Could you check a few things on this model? Use its own coordinates, in mm. Face numbers are marked on the shaded views. A direction names the side the tool comes from. Give positions to 0.01 mm unless a question says otherwise; leave off trailing zeros. Write each loop counter-clockwise with the first axis right and the second up, starting at its lowest first coordinate (ties: lowest second). Pieces come first, ordered by that corner, then holes. Notation, with made-up numbers: M -12.75,-30.5 L 3.25,-30.5 A22 cw 3.25,-5.5 Z; hole C -8.75,51 d8. An arc over 180 degrees is marked long. Use one line per item in the form item = value.
from build123d import *

# Parameters (mm, degrees)
F1_DEPTH = 63.5
F2_DEPTH = 25.4
F3_DEPTH = 7.9375
F5_R     = 6.35


with BuildPart() as f1:
    # F0 (on Front) → F1 (new body, symmetric)
    with BuildSketch(Plane.XZ):
        Polygon((22.225, 9.525), (-41.275, 9.525), (-41.275, -9.525), (41.275, -9.525), (41.275, 9.525), align=None)
    extrude(amount=F1_DEPTH, both=True)

    # F0 (on Front) → F2 (join, symmetric)
    with BuildSketch(Plane.XZ):
        with BuildLine():
            Line((22.225, 27.0002), (22.225, 9.525))
            Line((22.225, 9.525), (41.275, 9.525))
            Line((41.275, 9.525), (41.275, 27.0002))
            ThreePointArc((41.275, 27.0002), (45.92468, 38.22552), (57.15, 42.8752))
            Line((57.15, 42.8752), (60.325, 42.8752))
            Line((60.325, 42.8752), (60.325, 61.9252))
            Line((60.325, 61.9252), (57.15, 61.9252))
            add(Edge.make_bspline(
                [(54.083062, 61.790278), (55.113813, 61.853181), (56.136476, 61.898364), (57.15, 61.9252)],
                knots=[108.768433, 108.768433, 108.768433, 108.768433, 111.504536, 111.504536, 111.504536, 111.504536], degree=3))
            ThreePointArc((54.083062, 61.790278), (31.392783, 50.586667), (22.225, 27.0002))
        make_face()
    extrude(amount=F2_DEPTH, both=True)

    # F0 (on Front) → F3 (join, symmetric)
    with BuildSketch(Plane.XZ):
        with BuildLine():
            add(Edge.make_bspline(
                [(-41.275, 9.525), (-40.650702, 28.784269), (13.107559, 59.289674), (54.083062, 61.790278)],
                knots=[0, 0, 0, 0, 108.768433, 108.768433, 108.768433, 108.768433], degree=3))
            Line((-41.275, 9.525), (22.225, 9.525))
            Line((22.225, 9.525), (22.225, 27.0002))
            ThreePointArc((22.225, 27.0002), (31.392783, 50.586667), (54.083062, 61.790278))
        make_face()
    extrude(amount=F3_DEPTH, both=True)

    # F0 (on Front) → F4 (revolve)
    with BuildSketch(Plane.XZ):
        Polygon((60.325, 66.675), (60.325, 61.9252), (60.325, 42.8752), (60.325, 38.1), (85.725, 38.1), (85.616186, 66.675), align=None)
    revolve(axis=Axis((60.325, 0, 52.3875), (0, 0, 1)))

    # F5
    f5_edges = [f1.edges().sort_by_distance(p)[0] for p in [
        (41.275, -63.5, 0),
        (-41.275, -63.5, 0),
        (41.275, 63.5, 0),
        (-41.275, 63.5, 0),
    ]]
    fillet(f5_edges, radius=F5_R)


solid = f1.part
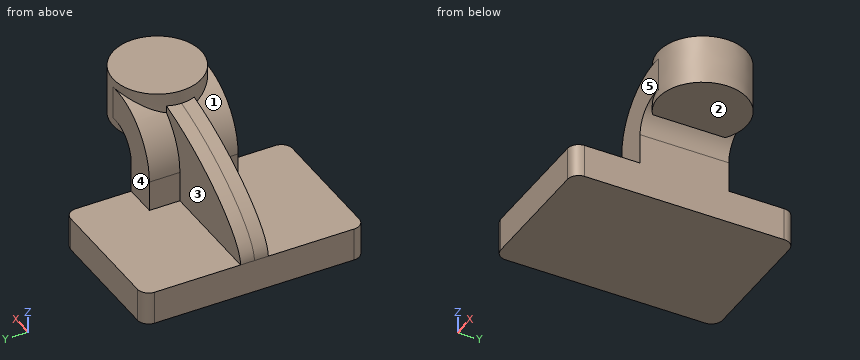
1) I want a section at A-A, the plane z = -1. Please give me the cut outline in (x, y) (3 decimals), plus the area to 3 significant figures.
Checked values:
outline = M -41.275,-57.15 A6.35 ccw -34.925,-63.5 L 34.925,-63.5 A6.35 ccw 41.275,-57.15 L 41.275,57.15 A6.35 ccw 34.925,63.5 L -34.925,63.5 A6.35 ccw -41.275,57.15 Z
area = 10,400 mm2
2) For the marked faces 1, 2, 3, 4 and 5, which set-ups out of +Z, -Z, +X, -X, +Y, -Y let a thin tool reach every point of the face, with its end or its side?
Checked values:
face_1 = +Z, -X, -Y
face_2 = -Z, +X, +Y, -Y
face_3 = +Z, -X, +Y
face_4 = +Z, +X, -X, +Y
face_5 = +Z, +X, -X, -Y
3) For pin 1 Ø8 at (y, z) = (-28, 10) entering from +X (3 decimals); pin 2 Ø5 at (x, z) = (14.5, 23) entering from -Y; pin 3 Ø1.5 at (x, z) = (71, 52) entering from +Y; pin 4 Ø19 at (y, z) = (-16.5, 16) entering from -X (3 decimals), each with a flat end and sliding along its axis, tell me the tip position at first contact or that it passes through.
Checked values:
pin_1 = 41.275
pin_2 = -7.94
pin_3 = 23.32
pin_4 = -41.275
4) If I drill on L1, parallel to Y at x = 39.5, z = 16.5; L2, parallel to Z at x = 14, y = -42.5 (3 decimals); L3, parallel to X at y = -24.5, z = 1 (3 decimals), over which ranges is the centre line in solid material (lowest first)?
Checked values:
L1 = -25.4 to 25.4
L2 = -9.525 to 9.525
L3 = -41.275 to 41.275
5) I want a section at B-B, the plane y = -31.5. Please give me the cut outline in (x, z) (3 decimals).
Checked values:
outline = M -41.275,-9.525 L 41.275,-9.525 L 41.275,9.525 L -41.275,9.525 Z
